```python
from build123d import *

# Parameters (mm, degrees)
F3_DEPTH = 96.774


with BuildPart() as f1:
    # F0 (on Right) → F1 (revolve)
    with BuildSketch(Plane.YZ):
        with BuildLine():
            Line((0, 40.851373), (0, 46.056358))
            ThreePointArc((0, 46.056358), (-46.056358, 0), (0, -46.056358))
            Line((0, -46.056358), (0, -40.851373))
            ThreePointArc((0, -40.851373), (-40.851373, 0), (0, 40.851373))
        make_face()
    revolve(axis=Axis((0, 0, 0), (0, 0, -1)))

    # F2 (on Right) → F3 (cut)
    with BuildSketch(Plane.YZ):
        with BuildLine():
            Line((16.023596, -3.039083), (21.411188, 4.818909))
            ThreePointArc((21.411188, 4.818909), (16.728984, 20.457276), (12.60009, 4.663802))
            Line((12.60009, 4.663802), (16.023596, -3.039083))
        make_face()
        Polygon((8.403815, -17.871678), (0, -8.289249), (-8.403815, -17.871678), (0, -17.871678), align=None)
        with BuildLine():
            Line((2.246329, -26.7301), (0, -29.67854))
            Line((0, -29.67854), (-2.246329, -26.7301))
            Line((-2.246329, -26.7301), (-5.966321, -29.564251))
            Line((-5.966321, -29.564251), (-10.19208, -24.017691))
            Line((-10.19208, -24.017691), (-13.962149, -26.889995))
            Line((-13.962149, -26.889995), (-15.514309, -20.464664))
            Line((-15.514309, -20.464664), (-18.094193, -24.017691))
            Line((-18.094193, -24.017691), (-19.936968, -19.911833))
            Line((-19.936968, -19.911833), (-21.411188, -23.228828))
            Line((-21.411188, -23.228828), (-24.359627, -15.304895))
            Line((-24.359627, -15.304895), (-27.069951, -16.313387))
            Line((-27.069951, -16.313387), (-27.676621, -13.093566))
            Line((-27.676621, -13.093566), (-31.614962, -13.835618))
            Line((-31.614962, -13.835618), (-31.614962, -8.855184))
            Line((-31.614962, -8.855184), (-34.549884, -7.550773))
            Line((-34.549884, -7.550773), (-38.670481, -5.719396))
            Line((-38.670481, -5.719396), (-37.627608, -11.435068))
            ThreePointArc((-37.627608, -11.435068), (-32.125537, -19.298328), (-25.221294, -25.96429))
            ThreePointArc((-25.221294, -25.96429), (-13.357962, -32.730942), (0, -35.57542))
            ThreePointArc((0, -35.57542), (13.357962, -32.730942), (25.221294, -25.96429))
            ThreePointArc((25.221294, -25.96429), (32.125537, -19.298328), (37.627608, -11.435068))
            Line((37.627608, -11.435068), (38.670481, -5.719396))
            Line((38.670481, -5.719396), (34.549884, -7.550773))
            Line((34.549884, -7.550773), (31.614962, -8.855184))
            Line((31.614962, -8.855184), (31.614962, -13.835618))
            Line((31.614962, -13.835618), (27.676621, -13.093566))
            Line((27.676621, -13.093566), (27.069951, -16.313387))
            Line((27.069951, -16.313387), (24.359627, -15.304895))
            Line((24.359627, -15.304895), (21.411188, -23.228828))
            Line((21.411188, -23.228828), (19.936968, -19.911833))
            Line((19.936968, -19.911833), (18.094193, -24.017691))
            Line((18.094193, -24.017691), (15.514309, -20.464664))
            Line((15.514309, -20.464664), (13.962149, -26.889995))
            Line((13.962149, -26.889995), (10.19208, -24.017691))
            Line((10.19208, -24.017691), (5.966321, -29.564251))
            Line((5.966321, -29.564251), (2.246329, -26.7301))
        make_face()
        with BuildLine():
            ThreePointArc((-12.60009, 4.663802), (-16.728984, 20.457276), (-21.411188, 4.818909))
            Line((-21.411188, 4.818909), (-16.023596, -3.039083))
            Line((-16.023596, -3.039083), (-12.60009, 4.663802))
        make_face()
    extrude(amount=-F3_DEPTH, mode=Mode.SUBTRACT)


solid = f1.part
```
The listing builds one solid part. Answer for the finished solid, in the listing's coordinates (mm). Give positions to 0.01 mm unless a question says otherwise; leave off trailing zeros. Order: outer loops, then holes, each group sorted by start corner. A loop starts at its lowest first (then second) coordinate and runs counter-clockwise, first axis right, second up. Notation, with made-up numbers: (34.5, -16) -> (76.5, -16) arc R15 ccw to (76.5, -10) -> close; hole circle Ø3 at (26, -27.5). An arc over 180 degrees is marked (long way). One line per item, written item: value.
1) Find section B-B, the plane y = -4.5. Determine the outline of the cut face in (x, z), plus the area to 3 significant figures.
Reported:
outline: (-43.83, -13.42) -> (-38.32, -13.42) arc R40.6 cw (long way) to (-20.42, -35.09) -> (-29.48, -35.09) arc R45.84 ccw (long way) to start; (-42.21, -17.87) arc R45.84 ccw to (-35.94, -28.45) -> (-28.97, -28.45) arc R40.6 cw to (-36.46, -17.87) -> close
area: 1,340 mm^2
2) Find section A-A, the plane z = 0. Determine the outline of the cut face in (x, y).
Reported:
outline: (-43.66, -14.67) -> (-38.13, -14.67) arc R40.85 cw to (-38.13, 14.67) -> (-43.66, 14.67) arc R46.06 ccw to start; (-42.35, -18.11) arc R46.06 ccw (long way) to (-42.35, 18.11) -> (-36.62, 18.11) arc R40.85 cw (long way) to (-36.62, -18.11) -> close
3) Find section C-C, the plane x = -15. Determine the outline of the cut face in (y, z), plus the area to 3 significant figures.
Reported:
outline: circle Ø87.09 at (0, 0); hole (-38.67, -5.72) -> (-37.63, -11.44) arc R49.95 ccw to (-34, -16.96) arc R38 ccw to (34, -16.96) arc R49.95 ccw to (37.63, -11.44) -> (38.67, -5.72) -> (37.48, -6.25) arc R38 ccw (long way) to (-37.48, -6.25) -> close
area: 1,400 mm^2
4) Find the intervals of material crossed by line 1 (X direction, y = 9.5, z = -13); line 2 (Y direction, x = -17.5, z = 27); line 3 (Y direction, x = 29, z = 9), in increasing order.
Reported:
line 1: x = -43.15 to -37.54, 37.54 to 43.15
line 2: y = -32.95 to -25.17, 25.17 to 32.95
line 3: y = -34.63 to -27.33, 27.33 to 34.63
5) Find section D-D, the plane z = 35.5. Determine the outline of the cut face in (x, y), plus the area to 3 significant figures.
Reported:
outline: circle Ø58.68 at (0, 0); hole circle Ø40.43 at (0, 0)
area: 1,420 mm^2
6) Flat-ended cylindrical pins translate along their axes: P1, Ø2.5, axis at x = -26.5, z = -10.5, coming from the -Y side; P2, Ø5, axis at y = 11, z = -17, coming from the +X side; P3, Ø1, axis at x = 25.5, y = 25.5, coming from the +Z side. Find the tip coordinate at first contact, or state that the pin passes through.
Reported:
P1: stops at y = -31.61
P2: stops at x = 42.5
P3: stops at z = 29.27
